Model file for the job. Use its own axes, mm. A direction names the side the tool comes from. Round coordinates to 2 decimals unless told otherwise and drop trailing zeros. Loops run counter-clockwise (first coordinate to the right, second up) from the corner with the lowest first, then second, coordinate; pieces in that order, holes last. Notation, with made-up numbers: (29.25, 32) -> (72.25, 32) arc R21 ccw to (72.25, 39) -> close; hole circle Ø10 at (-16, 15.25). An arc over 180 degrees is marked (long way). Use a Markdown table: item, result.
from build123d import *

# Parameters (mm, degrees)
SKETCH1_W           = 66
SKETCH1_H           = 85
BOSS_EXTRUDE1_DEPTH = 5
SKETCH5_W           = 22
SKETCH5_H           = 5
BOSS_EXTRUDE2_DEPTH = 7
SKETCH4_R           = 1.5
CUT_EXTRUDE2_DEPTH  = 10
SKETCH7_W           = 22
SKETCH7_H           = 5
BOSS_EXTRUDE3_DEPTH = 1
SKETCH8_W           = 22
SKETCH8_H           = 5
BOSS_EXTRUDE4_DEPTH = 1
SKETCH9_W           = 85
SKETCH9_H           = 5
BOSS_EXTRUDE5_DEPTH = 1
SKETCH10_W          = 85
SKETCH10_H          = 5
BOSS_EXTRUDE6_DEPTH = 1
SKETCH11_R          = 1.5
CUT_EXTRUDE3_DEPTH  = 10


with BuildPart() as part:
    # Sketch1 → Boss-Extrude1 (new body)
    with BuildSketch(Plane(origin=(0, 0, 0), x_dir=(1, 0, 0), z_dir=(0, 1, 0))):
        Rectangle(SKETCH1_W, SKETCH1_H)
    extrude(amount=BOSS_EXTRUDE1_DEPTH)

    # Sketch5 → Boss-Extrude2 (add)
    with BuildSketch(Plane.ZY.offset(33)):
        with Locations((0, 2.5)):
            Rectangle(SKETCH5_W, SKETCH5_H)
    boss_extrude2 = extrude(amount=BOSS_EXTRUDE2_DEPTH)

    # Mirror1: Boss-Extrude2 across plane
    add(boss_extrude2.mirror(Plane.ZY))

    # Sketch4 → Cut-Extrude2 (cut)
    with BuildSketch(Plane(origin=(0, 5, 0), x_dir=(1, 0, 0), z_dir=(0, 1, 0))):
        with Locations((-37.5, 7.5)):
            Circle(SKETCH4_R)
        with Locations((-21.5, 7.5)):
            Circle(SKETCH4_R)
        with Locations((-37.5, -7.5)):
            Circle(SKETCH4_R)
        with Locations((-21.5, -7.5)):
            Circle(SKETCH4_R)
        with Locations((21.5, -7.5)):
            Circle(SKETCH4_R)
        with Locations((37.5, -7.5)):
            Circle(SKETCH4_R)
        with Locations((21.5, 7.5)):
            Circle(SKETCH4_R)
        with Locations((37.5, 7.5)):
            Circle(SKETCH4_R)
    extrude(amount=-CUT_EXTRUDE2_DEPTH, mode=Mode.SUBTRACT)

    # Sketch7 → Boss-Extrude3 (add)
    with BuildSketch(Plane.ZY.offset(40)):
        with Locations((0, 2.5)):
            Rectangle(SKETCH7_W, SKETCH7_H)
    extrude(amount=BOSS_EXTRUDE3_DEPTH)

    # Sketch8 → Boss-Extrude4 (add)
    with BuildSketch(Plane(origin=(40, 0, 0), x_dir=(0, 0, -1), z_dir=(1, 0, 0))):
        with Locations((0, 2.5)):
            Rectangle(SKETCH8_W, SKETCH8_H)
    extrude(amount=BOSS_EXTRUDE4_DEPTH)

    # Sketch9 → Boss-Extrude5 (add)
    with BuildSketch(Plane.ZY.offset(33)):
        with Locations((0, 2.5)):
            Rectangle(SKETCH9_W, SKETCH9_H)
    extrude(amount=BOSS_EXTRUDE5_DEPTH)

    # Sketch10 → Boss-Extrude6 (add)
    with BuildSketch(Plane(origin=(33, 0, 0), x_dir=(0, 0, -1), z_dir=(1, 0, 0))):
        with Locations((0, 2.5)):
            Rectangle(SKETCH10_W, SKETCH10_H)
    extrude(amount=BOSS_EXTRUDE6_DEPTH)

    # Sketch11 → Cut-Extrude3 (cut)
    with BuildSketch(Plane(origin=(0, 5, 0), x_dir=(1, 0, 0), z_dir=(0, 1, 0))):
        with Locations((-20.5, -33.25)):
            Circle(SKETCH11_R)
        with Locations((-20.5, -19.75)):
            Circle(SKETCH11_R)
        with Locations((20.5, -33.25)):
            Circle(SKETCH11_R)
        with Locations((20.5, -19.75)):
            Circle(SKETCH11_R)
    extrude(amount=-CUT_EXTRUDE3_DEPTH, mode=Mode.SUBTRACT)


solid = part.part
Q1. Band-saw the part on D-D, the plane z = -7.5. Give the cut face in (x, y), plus the area to 3 significant figures.
Results list:
| item | result |
|---|---|
| outline | (-41, 0) -> (-39, 0) -> (-39, 5) -> (-41, 5) -> close; (-36, 0) -> (-23, 0) -> (-23, 5) -> (-36, 5) -> close; (-20, 0) -> (20, 0) -> (20, 5) -> (-20, 5) -> close; (23, 0) -> (36, 0) -> (36, 5) -> (23, 5) -> close; (39, 0) -> (41, 0) -> (41, 5) -> (39, 5) -> close |
| area | 350 mm² |
Q2. Band-saw the part on B-B, the plane y = 2.75. Give the number of separate pieces and of enclosed holes in the cut face, plus the area to 3 significant figures.
Results list:
| item | result |
|---|---|
| separate pieces | 1 |
| enclosed holes | 12 |
| area | 6,000 mm² |
Q3. Pull direction Z, two halves, no side cores. Call faces 4 (the face through (-22.7, 2.5, -6.6)), 5 (the face through (0, 2, -42.5)), 6 (the face through (-1, 5, 1)): released by +Z, released by -Z, zero draft, split by the parting line, or undercut.
Results list:
| item | result |
|---|---|
| face 4 | undercut |
| face 5 | released by -Z |
| face 6 | zero draft |
Q4. Flat gauge pins, fed straight in: pin 1 (2.5 mm diameter, centred on x = -38.5, y = 2.5, fed in from +Z); pin 2 (2.5 mm diameter, centred on x = 20.5, z = 33.25, fed in from +Y); pin 3 (1.5 mm diameter, centred on y = 2.5, z = 31.5, fed in from -X). Where does each tip first touch, or does it go through?
Results list:
| item | result |
|---|---|
| pin 1 | stops at z = 11 |
| pin 2 | passes through |
| pin 3 | stops at x = -34 |
Q5. Band-saw the part on A-A, the plane z = 19.75. Give the cut face in (x, y), plus the area to 3 significant figures.
Results list:
| item | result |
|---|---|
| outline | (-34, 0) -> (-22, 0) -> (-22, 5) -> (-34, 5) -> close; (-19, 0) -> (19, 0) -> (19, 5) -> (-19, 5) -> close; (22, 0) -> (34, 0) -> (34, 5) -> (22, 5) -> close |
| area | 310 mm² |
Q6. Tool access for faces 1 (the face through (34, 3, -27)), 2 (the face through (-34, 3, 27)), 3 (the face through (34, 3, 27)): list every direction of +Z, -Z, +X, -X, +Y, -Y with a clear straight run to the whole face (end or side of a thin tool).
Results list:
| item | result |
|---|---|
| face 1 | -Z, +X, +Y, -Y |
| face 2 | +Z, -X, +Y, -Y |
| face 3 | +Z, +X, +Y, -Y |
Q7. Band-saw the part on C-C, the plane x = -37.5. Give the cut face in (y, z).
Results list:
| item | result |
|---|---|
| outline | (0, -11) -> (5, -11) -> (5, -9) -> (0, -9) -> close; (0, -6) -> (5, -6) -> (5, 6) -> (0, 6) -> close; (0, 9) -> (5, 9) -> (5, 11) -> (0, 11) -> close |
Q8. Drill centre lines: L1, parallel to X at y = 3.75, z = -7.5; L2, parallel to X at y = 2.55, z = 19.75; L3, parallel to X at y = 1.5, z = 18.5. Where is each one in solid material? Low to high. Write a range as from..to.
Results list:
| item | result |
|---|---|
| L1 | x = -41..-39, -36..-23, -20..20, 23..36, 39..41 |
| L2 | x = -34..-22, -19..19, 22..34 |
| L3 | x = -34..-21.33, -19.67..19.67, 21.33..34 |
